from build123d import *

# Parameters (mm, degrees)
SKETCH1_R           = 1.4605
SKETCH1_R_2         = 12.7
BOSS_EXTRUDE1_DEPTH = 3.175
FILLET1_R           = 2.921


with BuildPart() as part:
    # Sketch1 → Boss-Extrude1 (new body)
    with BuildSketch(Plane(origin=(0, 0, 0), x_dir=(1, 0, 0), z_dir=(0, 1, 0))):
        with BuildLine():
            Line((5, -101.6), (5, 90.958222275))
            Line((5, 90.958222275), (57.514533832, 110.071949456))
            ThreePointArc((57.514533832, 110.071949456), (89.092337947, 97.415945766), (69.070568383, 124.919779784))
            Line((69.070568383, 124.919779784), (5, 101.6))
            Line((5, 101.6), (-5, 101.6))
            Line((-5, 101.6), (-5, -101.6))
            Line((-5, -101.6), (5, -101.6))
        make_face()
        with Locations(Location((0, -97.28, 0), (0, 0, 270))):
            Circle(SKETCH1_R, mode=Mode.SUBTRACT)
        with Locations(Location((0, 97.28, 0), (0, 0, 270))):
            Circle(SKETCH1_R, mode=Mode.SUBTRACT)
        with Locations(Location((75.12432492, 108.287220396, 0), (0, 0, 270))):
            Circle(SKETCH1_R_2, mode=Mode.SUBTRACT)
    extrude(amount=BOSS_EXTRUDE1_DEPTH)

    # Fillet1
    fillet1_edges = [part.edges().sort_by_distance(p)[0] for p in [
        (-5, 1.5875, 101.6),
        (-5, 1.5875, -101.6),
        (5, 1.5875, -101.6),
        (57.514533832, 1.5875, -110.071949456),
        (5, 1.5875, -90.958222275),
        (5, 1.5875, 101.6),
    ]]
    fillet(fillet1_edges, radius=FILLET1_R)


solid = part.part
CAD build for the part. Positions are in the model's coordinates, mm. A direction names the side the tool comes from. Coordinates: 2 decimals unless noted, no trailing zeros. Order: outer loops, then holes, each group sorted by start corner. A loop starts at its lowest first (then second) coordinate and runs counter-clockwise, first axis right, second up.
Item 1: Two-plate mould, pull along Z, no slides. Class faces 3 (the face through (78.939, 1.565, -96.174)), 4 (the face through (4, 0, -30)), 5 (the face through (89.85, 1.57, -98.47)): +Z half, -Z half, draft (parallel to the pull), parting line (faces both ways), or undercut.
Check sheet entries:
face 3: undercut
face 4: draft
face 5: parting line
Item 2: Band-saw the part on A-A on y = 1.8. List the corners of the cut face in (x, z).
Check sheet entries:
outline: (-5, -98.68) arc R2.92 ccw to (-2.08, -101.6) - (4.48, -101.6) arc R2.92 cw to (5.48, -101.78) - (69.07, -124.92) arc R17.7 ccw (long way) to (57.54, -106.25) arc R2.92 cw to (53.64, -108.66) - (6.92, -91.66) arc R2.92 cw to (5, -88.91) - (5, 98.68) arc R2.92 ccw to (2.08, 101.6) - (-2.08, 101.6) arc R2.92 ccw to (-5, 98.68) - close; hole circle Ø2.92 at (0, -97.28); hole circle Ø2.92 at (0, 97.28); hole circle Ø25.4 at (75.12, -108.29)
Item 3: 3-axis set-ups, long thin cutter, end or side, ignore diameter. For faces 1 (the face through (4, 3.175, -30)), 2 (the face through (29.95, 1.57, -100.04)): which of +Z, -Z, +X, -X, +Y, -Y reach the whole face in a straight line?
Check sheet entries:
face 1: +Z, -Z, +X, -X, +Y
face 2: +Z, +Y, -Y
Item 4: Band-saw the part on B-B on z = 12.5. List the corners of the cut face in (x, y) (3 decimals).
Check sheet entries:
outline: (-5, 0) - (5, 0) - (5, 3.175) - (-5, 3.175) - close
Item 5: Drill centre lines: L1, parallel to X at y = 1.8, z = 97.28; L2, parallel to X at y = 0.35, z = 20; L3, parallel to Z at x = 73, y = 0.4. Where is each one in solid material? Low to high.
Check sheet entries:
L1: x = -5 to -1.46, 1.46 to 5
L2: x = -5 to 5
L3: z = -125.86 to -120.81, -95.77 to -90.72
Item 6: Pin check, flat tip, straight feed: pin 1 Ø20.5 at (x, z) = (75.12, -108.29) entering from +Y (1 decimal). Stop position of the tip, or through.
Check sheet entries:
pin 1: passes through
